Design review of the part built by this model. Coordinates are the model's own, in mm. A direction names the side the tool comes from. Coordinates: 2 decimals unless noted, no trailing zeros. Write each loop counter-clockwise with the first axis right and the second up, starting at its lowest first coordinate (ties: lowest second). Pieces come first, ordered by that corner, then holes. Notation, with made-up numbers: M -40,80.25 L -27,80.25 A14 ccw -27,98.25 Z; hole C 7.25,6.25 d4. An arc over 180 degrees is marked long. One line per question, with ' | ' between items.
Autodesk Inventor part; units mm, degrees
ref_plane "YZ Plane" through (0, 0, 0) normal (1, 0, 0) x (0, 1, 0)
ref_plane "XZ Plane" through (0, 0, 0) normal (0, 1, 0) x (-1, 0, 0)
ref_plane "XY Plane" through (0, 0, 0) normal (0, 0, 1) x (1, 0, 0)
sketch "Sketch1" plane through (0, 0, 0) normal (0, 1, 0) x (-1, 0, 0)
  line L0 (0, -43.1) -> (0, 27.6) construction
  line L1 (-31.1, 0) -> (64.1, 0) construction
  arc A0 (17.5, 0) -> (-17.5, 0) centre (0, 0) ccw
  line L2 (17.5, 0) -> (17.5, -33)
  line L3 (17.5, 0) -> (50.5, 0) construction
  line L4 (-17.5, 0) -> (-17.5, -33)
  line L5 (-17.5, -33) -> (17.5, -33)
  circle A1 centre (0, 0) radius 5.05
  dimension "d0" = 35
  dimension "d1" = 33
  dimension "d2" = 90
  dimension "d3" = 10.1
extrude "Extrusion1" add sketch "Sketch1" along normal blind 3
sketch "Sketch5" plane through (0, 0, 0) normal (0, -1, 0) x (1, 0, 0)
  circle A0 centre (0, 0) radius 5.05 construction
  arc A1 (17.5, 0) -> (-17.5, 0) centre (0, 0) ccw construction
  line L0 (-17.5, -33) -> (-17.5, 0) construction
  line L1 (17.5, -33) -> (-17.5, -33) construction
  line L2 (17.5, 0) -> (17.5, -33) construction
  line L3 (17.5, 0) -> (17.5, -33)
  line L4 (-17.5, -33) -> (-17.5, 0)
  line L5 (17.5, -33) -> (-17.5, -33)
  line L6 (-17.5, -33) -> (-17.5, -30)
  line L7 (-17.5, -30) -> (17.5, -30)
  line L8 (17.5, -30) -> (17.5, -33)
  dimension "d11" = 3
extrude "Extrusion4" add sketch "Sketch5" against normal blind 70
sketch "Sketch6" plane through (0, 70, 0) normal (0, 1, 0) x (1, 0, 0)
  line L0 (17.5, 0) -> (17.5, 33)
  arc A0 (-17.5, 0) -> (17.5, 0) centre (0, 0) ccw
  line L1 (-17.5, 33) -> (-17.5, 0)
  line L2 (17.5, 33) -> (-17.5, 33)
  circle A1 centre (0, 0) radius 5.05
extrude "Extrusion5" add sketch "Sketch6" against normal blind 3
properties part number "steering_kingpin_bracket" material "Steel, Mild"
1. Take a section at C-C (y = 54). Write out the cut boundary in (x, z), then the cut area to 3 significant figures.
Answer sheet:
outline: M -17.5,-33 L 17.5,-33 L 17.5,-30 L -17.5,-30 Z | area: 105 mm^2
2. Take a section at B-B (z = -14.5). Write out the cut boundary in (x, y).
Answer sheet:
outline: M -17.5,0 L 17.5,0 L 17.5,3 L -17.5,3 Z; M -17.5,67 L 17.5,67 L 17.5,70 L -17.5,70 Z
3. Insertion check: pin 1 Ø8 at (x, z) = (6, -17) entering from -Y; pin 2 Ø1.5 at (x, y) = (-1.5, 10) entering from +Z. Each pin has a flat end and moves straight along its axis. Give the tip position at first contact, or say it passes through.
Answer sheet:
pin 1: y = 0 | pin 2: z = -30
4. Draft analysis for pull direction Y (two halves, no side actions). For faces 3 (the face through (0, 0, -7)), 4 (the face through (4.817, 68.521, -1.517)), 5 (the face through (0, 3, -6)), 6 (the face through (0, 70, -8)), state which applies: pulls with the +Y half, pulls with the -Y half, needs draft (parallel to the pull), parting line crosses it, or undercut.
Answer sheet:
face 3: pulls with the -Y half | face 4: needs draft | face 5: undercut | face 6: pulls with the +Y half
5. To check wall thickness, follow line 1 along Z through (x, y) = (0, 69); line 2 along Y through (x, z) = (12.5, -25); line 3 along X through (y, z) = (68.3, 0). State the ranges of each line that lie inside material, in increasing order. Write a range as [from, to].
Answer sheet:
line 1: [-33, -5.05], [5.05, 17.5] | line 2: [0, 3], [67, 70] | line 3: [-17.5, -5.05], [5.05, 17.5]
6. Tool access review of faces 1 (the face through (0, 67, -7)), 2 (the face through (-4.817, 1.479, -1.517)): name each direction out of +Z, -Z, +X, -X, +Y, -Y from which nothing blocks a thin tool from reaching the whole face with its end or side.
Answer sheet:
face 1: +Z, +X, -X | face 2: +Y, -Y
7. Take a section at D-D (x = 6.5). Write out the cut boundary in (y, z), then the cut area to 3 significant figures.
Answer sheet:
outline: M 0,-33 L 70,-33 L 70,16.25 L 67,16.25 L 67,-30 L 3,-30 L 3,16.25 L 0,16.25 Z | area: 487 mm^2
8. Take a section at A-A (x = 0). Write out the cut boundary in (y, z), then the cut area to 3 significant figures.
Answer sheet:
outline: M 0,-33 L 70,-33 L 70,-5.05 L 67,-5.05 L 67,-30 L 3,-30 L 3,-5.05 L 0,-5.05 Z; M 0,5.05 L 3,5.05 L 3,17.5 L 0,17.5 Z; M 67,5.05 L 70,5.05 L 70,17.5 L 67,17.5 Z | area: 434 mm^2
